Verification items for the finished model (mm, model axes). A direction names the side the tool comes from. Give positions to 0.01 mm unless a question says otherwise; leave off trailing zeros. Order: outer loops, then holes, each group sorted by start corner. A loop starts at its lowest first (then second) coordinate and runs counter-clockwise, first axis right, second up. Notation, with made-up numbers: (-23, -2) - (0, -2) arc R30 cw to (0, 22) - close; hole circle Ø7 at (46.5, 39.5). An arc over 180 degrees is marked (long way). Answer as a JSON object with one key per item and string values.
Autodesk Inventor part; units mm, degrees
ref_plane "YZ Plane" through (0, 0, 0) normal (1, 0, 0) x (0, 1, 0)
ref_plane "XZ Plane" through (0, 0, 0) normal (0, 1, 0) x (-1, 0, 0)
ref_plane "XY Plane" through (0, 0, 0) normal (0, 0, 1) x (1, 0, 0)
sketch "Sketch1" plane through (0, 0, 0) normal (0, 1, 0) x (-1, 0, 0)
  circle A0 centre (0, 0) radius 45.5
  dimension "d0" = 91
extrude "Extrusion1" add sketch "Sketch1" along normal blind 7
sketch "Sketch5" plane through (0, 7, 0) normal (0, 1, 0) x (1, 0, 0)
  circle A0 centre (0, 0) radius 6
  dimension "d27" = 12
extrude "Extrusion5" add sketch "Sketch5" along normal blind 2
sketch "Sketch7" plane through (0, 0, 0) normal (0, -1, 0) x (1, 0, 0)
  circle A0 centre (0, 0) radius 45.5
  line L0 (0, 0) -> (33, 0)
  circle A1 centre (33, 0) radius 2
  dimension "d37" = 4
  dimension "d38" = 33
extrude "Extrusion7" cut sketch "Sketch7" against normal blind 10 contours A1
pattern_circular "Circular Pattern1" count 12 over 360 about axis through (0, 0, 0) along (0, -1, 0) of "Extrusion7"
sketch "Sketch8" plane through (0, 0, 0) normal (0, -1, 0) x (1, 0, 0)
  circle A0 centre (-13.726, 35.2198) radius 1.5
  circle A1 centre (13.726, -35.2198) radius 1.5
  circle A2 centre (-16.5, 28.5788) radius 2
  line L0 (-13.726, 35.2198) -> (13.726, -35.2198) construction
  point P0 (0, 0)
  point P1 (0, 0)
  dimension "d46" = 3
  dimension "d48" = 3
  dimension "d51" = 6.641
  dimension "d52" = 75.6
extrude "Extrusion8" cut sketch "Sketch8" against normal blind 10 contours A0 | A1
properties part number "bay container 12 bottom"
(1) Section check B-B (x = -33). Record the cut outline in (y, z), then the cut area to 3 significant figures.
Computed values:
{"outline": "(0, -31.32) - (7, -31.32) - (7, -2) - (0, -2) - close; (0, 2) - (7, 2) - (7, 31.32) - (0, 31.32) - close", "area": "411 mm²"}
(2) Gauge pin test, flat ends, axial feed: pin 1 Ø1.5 at (x, z) = (36.5, 22) entering from +Y; pin 2 Ø3 at (x, z) = (33, 0) entering from -Y; pin 3 Ø3 at (y, z) = (2, 17) entering from -X. Record the tip position at first contact, or that the pin passes through.
Computed values:
{"pin 1": "stops at y = 7", "pin 2": "passes through", "pin 3": "stops at x = -42.78"}
(3) Release check for a two-part mould opening along X. For faces 1 (the cylindrical face through (36.107, 3.451, 27.686)), 2 (the flat face through (0, 9, 0)), 3 (the cylindrical face through (18.087, 3.451, 29.796)) record: pulls with the +X half, pulls with the -X half, needs draft (parallel to the pull), parting line crosses it, or undercut.
Computed values:
{"face 1": "parting line crosses it", "face 2": "needs draft", "face 3": "undercut"}
(4) Section check D-D (x = 40). Record the cut outline in (y, z), then the cut area to 3 significant figures.
Computed values:
{"outline": "(0, -21.69) - (7, -21.69) - (7, 21.69) - (0, 21.69) - close", "area": "304 mm²"}
(5) Section check A-A (z = 0). Record the cut outline in (x, y).
Computed values:
{"outline": "(-45.5, 0) - (-35, 0) - (-35, 7) - (-45.5, 7) - close; (-31, 0) - (31, 0) - (31, 7) - (6, 7) - (6, 9) - (-6, 9) - (-6, 7) - (-31, 7) - close; (35, 0) - (45.5, 0) - (45.5, 7) - (35, 7) - close"}
(6) Access from +Z, -Z, +X, -X, +Y, -Y to the whole of each face (thin tool, end or side, straight path). Record for faces 4 (the cylindrical face through (-6, 8, 0)), 5 (the cylindrical face through (-0.766, 3.451, -34.847)).
Computed values:
{"face 4": "+Y", "face 5": "+Y, -Y"}
(7) Section check C-C (y = 3.5). Count the separate pieces of the cut face and the enclosed holes in it, then the cut area to 3 significant figures.
Computed values:
{"separate pieces": "1", "enclosed holes": "14", "area": "6,340 mm²"}
(8) Material ranges on line 1 along Z through (x, y) = (0, 2.25); line 2 along Z through (x, y) = (-27, 2.25); line 3 along X through (y, z) = (5.25, -29), recorded low to high. Write a range as [from, to].
Computed values:
{"line 1": "z = [-45.5, -35], [-31, 31], [35, 45.5]", "line 2": "z = [-36.62, -17.73], [-15.27, 15.27], [17.73, 36.62]", "line 3": "x = [-35.06, -18.46], [-14.54, 14.54], [18.46, 35.06]"}
